from build123d import *

# Parameters (mm, degrees)
EXTRUDE_1_DEPTH     = 6
CUT_EXTRUDE_1_DEPTH = 10.5
SKETCH_3_R          = 1.5
CUT_EXTRUDE_2_DEPTH = 10.5


with BuildPart() as part:
    # 草图1 → 凸台-拉伸1 (new body)
    with BuildSketch(Plane.XY):
        with BuildLine():
            Line((12, 4), (12, -4))
            Line((12, -4), (3.774917218, -4))
            ThreePointArc((3.774917218, -4), (0, -5.5), (-3.774917218, -4))
            Line((-3.774917218, -4), (-12, -4))
            Line((-12, -4), (-12, -1))
            Line((-12, -1), (-3.872983346, -1))
            ThreePointArc((-3.872983346, -1), (4, 0), (-3.872983346, 1))
            Line((-3.872983346, 1), (-12, 1))
            Line((-12, 1), (-12, 4))
            Line((-12, 4), (-3.774917218, 4))
            ThreePointArc((-3.774917218, 4), (0, 5.5), (3.774917218, 4))
            Line((3.774917218, 4), (12, 4))
        make_face()
    extrude(amount=EXTRUDE_1_DEPTH)

    # 草图2 → 切除-拉伸1 (cut, through all)
    with BuildSketch(Plane.XZ.offset(4)):
        with BuildLine():
            ThreePointArc((-9, 0), (-11.121320344, 0.878679656), (-12, 3))
            Line((-12, 3), (-12, 0))
            Line((-12, 0), (-9, 0))
        make_face()
        with BuildLine():
            Line((-9, 6), (-12, 6))
            Line((-12, 6), (-12, 3))
            ThreePointArc((-12, 3), (-11.121320344, 5.121320344), (-9, 6))
        make_face()
        with BuildLine():
            Line((12, 0), (12, 3))
            ThreePointArc((12, 3), (11.121320344, 0.878679656), (9, 0))
            Line((9, 0), (12, 0))
        make_face()
        with BuildLine():
            Line((12, 6), (9, 6))
            ThreePointArc((9, 6), (11.121320344, 5.121320344), (12, 3))
            Line((12, 3), (12, 6))
        make_face()
    extrude(amount=-CUT_EXTRUDE_1_DEPTH, mode=Mode.SUBTRACT)

    # 草图3 → 切除-拉伸2 (cut, through all)
    with BuildSketch(Plane.XZ.offset(4)):
        with Locations((-9, 3)):
            Circle(SKETCH_3_R)
        with Locations((9, 3)):
            Circle(SKETCH_3_R)
    extrude(amount=-CUT_EXTRUDE_2_DEPTH, mode=Mode.SUBTRACT)


solid = part.part
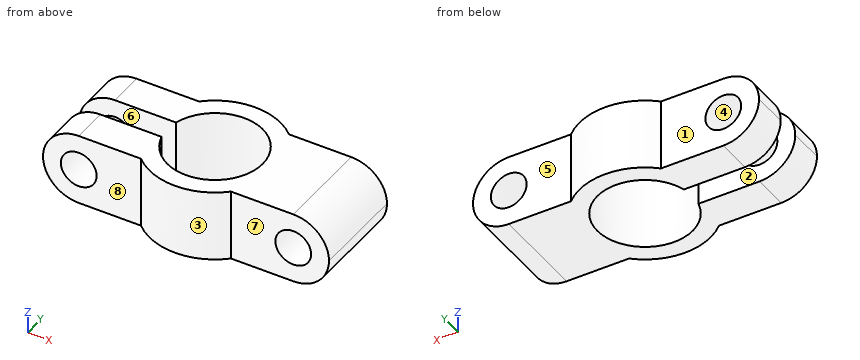
Input: part model. Units: mm. Frame: model coordinates. Face numbers are marked on the shaded views. A direction names the side the tool comes from. Give positions to 0.01 mm unless a question says otherwise; leave off trailing zeros. Write each loop counter-clockwise with the first axis right and the second up, starting at its lowest first coordinate (ties: lowest second). Pieces come first, ordered by that corner, then holes. Notation, with made-up numbers: M 40.5,-12.5 L 91.5,-12.5 A21 cw 91.5,21.5 Z; hole C 9,29.5 d1. An arc over 180 degrees is marked long. Use one line per item in the form item = value.
1. Cut plane C-C on y = 0. Return loops of the section in (x, z).
Outcome:
outline = M 4,0 L 9,0 A3 ccw 9,6 L 4,6 Z; hole C 9,3 d3
2. Reachability of the marked faces 5, 6, 7 and 8 from +Z, -Z, +X, -X, +Y, -Y: full face, straight path, thin tool, end or side. Return the list, or none.
Outcome:
face_5 = +Z, -Z, +X, +Y
face_6 = +Z, -Z, -X
face_7 = +Z, -Z, +X, -Y
face_8 = +Z, -Z, -X, -Y
3. Cut plane A-A on x = 0. Return loops of the section in (y, z), and give its area (3 significant figures).
Outcome:
outline = M -5.5,0 L -4,0 L -4,6 L -5.5,6 Z; M 4,0 L 5.5,0 L 5.5,6 L 4,6 Z
area = 18.0 mm²
4. Mould query, pull axis Y, two halves, no side actions, for the marked faces 1, 2, 3 and 4. Classes: released by +Y, released by -Y, zero draft, split by the parting line, or undercut.
Outcome:
face_1 = released by +Y
face_2 = undercut
face_3 = released by -Y
face_4 = zero draft
5. Ray query, L1, parallel to Z at x = -9, y = 2.25; L2, parallel to Y at x = -5, z = 1.75; L3, parallel to Y at x = 10.5, z = 1.25. Return the intervals inside material, ascending.
Outcome:
L1 = 0 to 1.5, 4.5 to 6
L2 = -4 to -1, 1 to 4
L3 = -4 to 4
6. First-contact query: P1, Ø1.5, axis at x = -7, z = 2.5, coming from the -Y side; P2, Ø3, axis at y = -3.5, z = 5, coming from the -X side; P3, Ø3, axis at x = 7, z = 2.5, coming from the +Y side. Flat tips, straight axial feed; report the tip coordinate or a pass-through.
Outcome:
P1 = -4
P2 = -11.96
P3 = 4
7. Cut plane B-B on y = -2.5. Return loops of the section in (x, z).
Outcome:
outline = M -9,0 L -3.12,0 L -3.12,6 L -9,6 A3 ccw Z; M 3.12,0 L 9,0 A3 ccw 9,6 L 3.12,6 Z; hole C -9,3 d3; hole C 9,3 d3
8. Cut plane D-D on x = -6.5. Return loops of the section in (y, z).
Outcome:
outline = M -4,0 L -1,0 L -1,6 L -4,6 Z; M 1,0 L 4,0 L 4,6 L 1,6 Z
